Geometry: final body of the model. Coordinates: model frame, mm. Coordinates: 2 decimals unless noted, no trailing zeros. Loops run counter-clockwise (first coordinate to the right, second up) from the corner with the lowest first, then second, coordinate; pieces in that order, holes last. Notation, with made-up numbers: M 49.5,-39 L 108.5,-39 A14 ccw 108.5,-28 Z; hole C 0.5,-8.75 d5. An arc over 180 degrees is marked long. Write item = value, one per line. Start each with the question number.
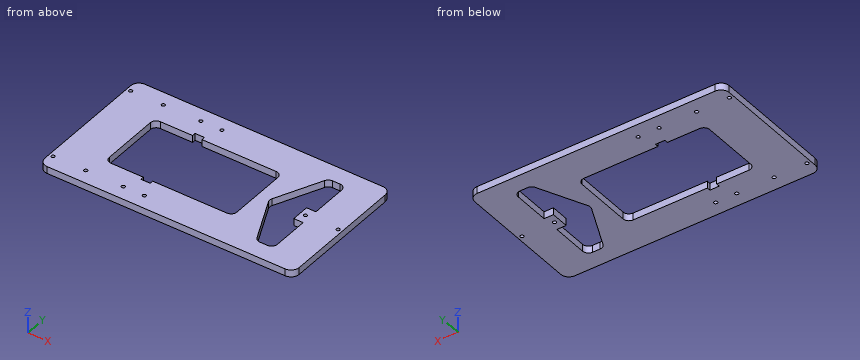
```python
from build123d import *

# Parameters (mm, degrees)
SKETCH1_W           = 218
SKETCH1_H           = 117.2
SKETCH1_R           = 1.5
BOSS_EXTRUDE1_DEPTH = 6
SKETCH2_R           = 1.5
CUT_EXTRUDE1_DEPTH  = 6
FILLET1_R           = 7
SKETCH3_W           = 109.333333333
SKETCH3_H           = 59.2
CUT_EXTRUDE2_DEPTH  = 10
FILLET3_R           = 5
CUT_EXTRUDE3_DEPTH  = 10
FILLET4_R           = 5
SKETCH5_W           = 8
SKETCH5_H           = 65.2
CUT_EXTRUDE4_DEPTH  = 10


with BuildPart() as part:
    # Sketch1 → Boss-Extrude1 (new body)
    with BuildSketch(Plane.XY):
        with Locations((-150.609177744, 197.743600407)):
            Rectangle(SKETCH1_W, SKETCH1_H)
        with Locations((-256.109177744, 244.343600407)):
            Circle(SKETCH1_R, mode=Mode.SUBTRACT)
        with Locations((-256.109177744, 151.143600407)):
            Circle(SKETCH1_R, mode=Mode.SUBTRACT)
        with Locations((-45.109177744, 197.743600407)):
            Circle(SKETCH1_R, mode=Mode.SUBTRACT)
        with Locations((-73.109177744, 197.743600407)):
            Circle(SKETCH1_R, mode=Mode.SUBTRACT)
        with Locations((-228.109177744, 244.343600407)):
            Circle(SKETCH1_R, mode=Mode.SUBTRACT)
        with Locations((-228.109177744, 151.143600407)):
            Circle(SKETCH1_R, mode=Mode.SUBTRACT)
    extrude(amount=BOSS_EXTRUDE1_DEPTH)

    # Sketch2 → Cut-Extrude1 (cut)
    with BuildSketch(Plane.XY.offset(6)):
        with Locations((-195.942511077, 151.143600407)):
            Circle(SKETCH2_R)
        with Locations((-177.942511077, 151.143600407)):
            Circle(SKETCH2_R)
        with Locations((-195.942511077, 244.343600407)):
            Circle(SKETCH2_R)
        with Locations((-177.942511077, 244.343600407)):
            Circle(SKETCH2_R)
    extrude(amount=-CUT_EXTRUDE1_DEPTH, mode=Mode.SUBTRACT)

    # Fillet1
    fillet1_edges = [part.edges().sort_by_distance(p)[0] for p in [
        (-259.609177744, 256.343600407, 3),
        (-41.609177744, 256.343600407, 3),
        (-41.609177744, 139.143600407, 3),
        (-259.609177744, 139.143600407, 3),
    ]]
    fillet(fillet1_edges, radius=FILLET1_R)

    # Sketch3 → Cut-Extrude2 (cut)
    with BuildSketch(Plane(origin=(0, 0, 0), x_dir=(-1, 0, 0), z_dir=(0, 0, -1))):
        with Locations((168.942511078, 197.743600407)):
            Rectangle(SKETCH3_W, SKETCH3_H)
    extrude(amount=-CUT_EXTRUDE2_DEPTH, mode=Mode.SUBTRACT)

    # Fillet3
    fillet3_edges = [part.edges().sort_by_distance(p)[0] for p in [
        (-114.275844411, 227.343600407, 3),
        (-223.609177744, 227.343600407, 3),
        (-223.609177744, 168.143600407, 3),
        (-114.275844411, 168.143600407, 3),
    ]]
    fillet(fillet3_edges, radius=FILLET3_R)

    # Sketch4 → Cut-Extrude3 (cut)
    with BuildSketch(Plane(origin=(0, 0, 0), x_dir=(-1, 0, 0), z_dir=(0, 0, -1))):
        Polygon((84.298987117, 241.343600407), (69.597266226, 241.343600407), (69.597266226, 205.418600407), (77.609177744, 205.418600407), (77.609177744, 190.068600407), (69.597266226, 190.068600407), (69.597266226, 154.143600407), (84.298987117, 154.143600407), (104.275844411, 197.743600407), align=None)
    extrude(amount=-CUT_EXTRUDE3_DEPTH, mode=Mode.SUBTRACT)

    # Fillet4
    fillet4_edges = [part.edges().sort_by_distance(p)[0] for p in [
        (-69.597266226, 241.343600407, 3),
        (-84.298987117, 241.343600407, 3),
        (-104.275844411, 197.743600407, 3),
        (-84.298987117, 154.143600407, 3),
        (-69.597266226, 154.143600407, 3),
    ]]
    fillet(fillet4_edges, radius=FILLET4_R)

    # Sketch5 → Cut-Extrude4 (cut)
    with BuildSketch(Plane(origin=(0, 0, 0), x_dir=(-1, 0, 0), z_dir=(0, 0, -1))):
        with Locations((186.942511077, 197.743600407)):
            Rectangle(SKETCH5_W, SKETCH5_H)
    extrude(amount=-CUT_EXTRUDE4_DEPTH, mode=Mode.SUBTRACT)


solid = part.part
```
Item 1: Section query D-D (z = 1.25). Count the separate pieces of the cut face and the enclosed holes in it, plus the area to 3 significant figures.
Item 2: Section query A-A (x = -213). Return the cut outline in (y, z).
Item 3: Section query C-C (y = 163). Return the cut outline in (x, z), plus the area to 3 significant figures.
Item 4: First-contact query: pin 1 (3.5 mm diameter, centred on x = -256.11, y = 151.14, fed in from -Z); pin 2 (1.8 mm diameter, centred on x = -256.11, y = 244.34, fed in from +Z). Flat tips, straight axial feed; report the tip coordinate or a pass-through.
Item 5: Section query B-B (y = 202). Return the cut outline in (x, z).
Item 6: Line query: line 1 (Y direction, x = -228, z = 4); line 2 (X direction, y = 151, z = 4); line 3 (Y direction, x = -163, z = 3.75). Output: solid intervals per line, ascending. Write a range as from..to.
Verdict:
q1.separate_pieces = 1
q1.enclosed_holes = 12
q1.area = 16,900 mm2
q2.outline = M 139.14,0 L 168.14,0 L 168.14,6 L 139.14,6 Z; M 227.34,0 L 256.34,0 L 256.34,6 L 227.34,6 Z
q3.outline = M -259.61,0 L -88.36,0 L -88.36,6 L -259.61,6 Z; M -69.6,0 L -41.61,0 L -41.61,6 L -69.6,6 Z
q3.area = 1,200 mm2
q4.pin_1 = 0
q4.pin_2 = through
q5.outline = M -259.61,0 L -223.61,0 L -223.61,6 L -259.61,6 Z; M -114.28,0 L -102.33,0 L -102.33,6 L -114.28,6 Z; M -77.61,0 L -41.61,0 L -41.61,6 L -77.61,6 Z
q6.line_1 = 139.14..149.65, 152.64..242.85, 245.84..256.34
q6.line_2 = -259.61..-257.6, -254.62..-229.6, -226.62..-197.44, -194.45..-179.44, -176.45..-41.61
q6.line_3 = 139.14..168.14, 227.34..256.34
